Source: CAD feature listing. Evaluate the final solid. Frame: model axes, mm. A direction names the side the tool comes from. Give positions to 0.01 mm unless a question says otherwise; leave off trailing zeros. Answer in a Markdown table with one row per item.
```python
from build123d import *

# Parameters (mm, degrees)
F0_W     = 1066.8
F0_H     = 993.775
F1_DEPTH = 457.2
F2_W     = 1066.8
F2_H     = 3.175
F2_H_2   = 41.148
F3_DEPTH = 25.4


with BuildPart() as f1:
    # F0 (on Front) → F1 (new body)
    with BuildSketch(Plane.XZ):
        Rectangle(F0_W, F0_H)
    extrude(amount=F1_DEPTH)

    # F2 (on face) → F3 (cut)
    with BuildSketch(Plane.XZ.offset(457.2)):
        with Locations((0, 180.975)):
            Rectangle(F2_W, F2_H)
        with Locations((0, -139.827)):
            Rectangle(F2_W, F2_H)
        with Locations((0, -476.3135)):
            Rectangle(F2_W, F2_H_2)
    extrude(amount=-F3_DEPTH, mode=Mode.SUBTRACT)


solid = f1.part
```
(1) First-contact query: pin 1 Ø1.6 at (x, z) = (29.5, -139.5) entering from -Y; pin 2 Ø20.5 at (x, y) = (55.5, -443.5) entering from -Z. Flat tips, straight axial feed; report the tip coordinate or a pass-through.
A:
| item | result |
|---|---|
| pin 1 | stops at y = -431.8 |
| pin 2 | stops at z = -455.74 |
(2) Pull-direction query (Z, two-part tool) for faces 1 (the flat face through (-7, -445, -455.739)), 2 (the flat face through (-533.4, -225, -7)), 3 (the flat face through (-7, -445, -138.24)); classes: +Z half, -Z half, draft (parallel to the pull), parting line (faces both ways), or undercut.
A:
| item | result |
|---|---|
| face 1 | -Z half |
| face 2 | draft |
| face 3 | undercut |
(3) Access query for faces 4 (the flat face through (-7, -213, -496.888)), 5 (the flat face through (-7, -445, 179.388)), 6 (the flat face through (-7, -431.8, -476)). Directions: +Z, -Z, +X, -X, +Y, -Y. A direction counts if a zero-diameter tool reaches every point of the face in a straight line with its end or side. Return the directions, or none.
A:
| item | result |
|---|---|
| face 4 | -Z, +X, -X, +Y, -Y |
| face 5 | +X, -X, -Y |
| face 6 | -Z, +X, -X, -Y |
